For this review, take the finished solid that the model builds, in its own axes (mm). Give positions to 0.01 mm unless a question says otherwise; leave off trailing zeros. Order: outer loops, then holes, each group sorted by start corner. A loop starts at its lowest first (then second) coordinate and runs counter-clockwise, first axis right, second up. Notation, with made-up numbers: M 32.25,51 L 63.25,51 A15 cw 63.25,69 Z; hole C 0,44 d10. An arc over 180 degrees is marked long. Answer as CSV lines item,"result". Start each with the question number.
1. We need section B-B, the plane z = 8. Give the boundary of the cut face in (x, y), and give its area (3 significant figures).
2. For line 1 along Z through (x, y) = (30, 0.5); line 2 along X through (y, z) = (2.1, 31.5); line 3 along X through (y, z) = (2.35, -31.5), list the stretches that pass through material, from the lowest coordinate up.
3. We need section C-C, the plane z = -16.5. Give the boundary of the cut face in (x, y).
4. Clearance check with flat-ended pins moving along their axes: P1, Ø1.5, axis at y = 1.5, z = -32.5, coming from the +X side; P2, Ø1.8, axis at x = 43.75, z = 31.5, coming from the +Y side; P3, Ø1, axis at x = -29, y = 2, coming from the -Z side; P4, Ø0.9, axis at y = 1.5, z = 0.5, coming from the +X side. State where each tip first meets the part, or that it passes through.
5. We need section D-D, the plane y = 1.3. State how many separate pieces and enclosed holes the cut face has, and give its area (3 significant figures).
6. We need section A-A, the plane x = -43.25. Give the boundary of the cut face in (y, z).
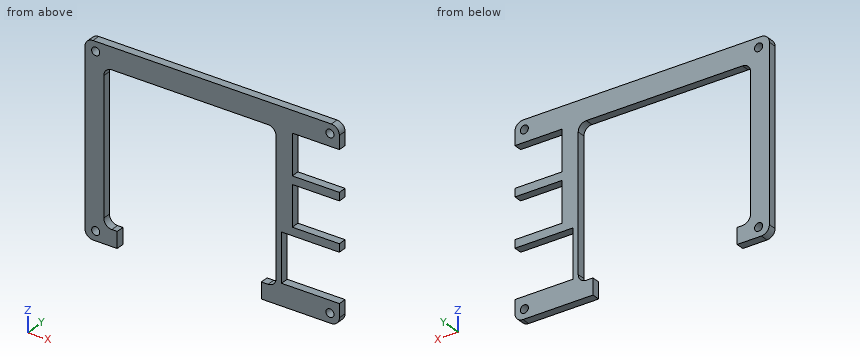
from build123d import *

# Parameters (mm, degrees)
SKETCH1_W           = 94.5
SKETCH1_H           = 70
BOSS_EXTRUDE1_DEPTH = 3
SKETCH3_R           = 1.5
CUT_EXTRUDE2_DEPTH  = 59.877521177
FILLET2_R           = 3
SKETCH5_W           = 64
SKETCH5_H           = 56
SKETCH5_W_2         = 53.5
SKETCH5_H_2         = 6
SKETCH5_W_3         = 21.5
SKETCH5_H_3         = 18
SKETCH5_W_4         = 17.5
SKETCH5_H_4         = 15
CUT_EXTRUDE3_DEPTH  = 59.877521177
FILLET3_R           = 3


with BuildPart() as part:
    # Sketch1 → Boss-Extrude1 (new body)
    with BuildSketch(Plane(origin=(0, 0, 0), x_dir=(1, 0, 0), z_dir=(0, 1, 0))):
        Rectangle(SKETCH1_W, SKETCH1_H)
    extrude(amount=BOSS_EXTRUDE1_DEPTH)

    # Sketch3 → Cut-Extrude2 (cut, through all)
    with BuildSketch(Plane(origin=(0, 3, 0), x_dir=(1, 0, 0), z_dir=(0, 1, 0))):
        with Locations(Location((43.75, 31.5, 0), (0, 0, 270))):
            Circle(SKETCH3_R)
        with Locations(Location((-43.25, 31.5, 0), (0, 0, 270))):
            Circle(SKETCH3_R)
        with Locations(Location((-43.25, -31.5, 0), (0, 0, 270))):
            Circle(SKETCH3_R)
        with Locations(Location((43.75, -31.5, 0), (0, 0, 270))):
            Circle(SKETCH3_R)
    extrude(amount=-CUT_EXTRUDE2_DEPTH, mode=Mode.SUBTRACT)

    # Fillet2
    fillet2_edges = [part.edges().sort_by_distance(p)[0] for p in [
        (47.25, 1.5, 35),
        (-47.25, 1.5, 35),
        (-47.25, 1.5, -35),
        (47.25, 1.5, -35),
    ]]
    fillet(fillet2_edges, radius=FILLET2_R)

    # Sketch5 → Cut-Extrude3 (cut, through all)
    with BuildSketch(Plane(origin=(0, 3, 0), x_dir=(1, 0, 0), z_dir=(0, 1, 0))):
        with Locations((-8.25, 1)):
            Rectangle(SKETCH5_W, SKETCH5_H)
        with Locations((-8.5, 32)):
            Rectangle(SKETCH5_W_2, SKETCH5_H_2)
        with Locations((36.5, 18)):
            Rectangle(SKETCH5_W_3, SKETCH5_H_3)
        with Locations((38.5, -1.5)):
            Rectangle(SKETCH5_W_4, SKETCH5_H_4)
        with Locations((38.5, -19.5)):
            Rectangle(SKETCH5_W_4, SKETCH5_H_4)
    extrude(amount=-CUT_EXTRUDE3_DEPTH, mode=Mode.SUBTRACT)

    # Fillet3
    fillet3_edges = [part.edges().sort_by_distance(p)[0] for p in [
        (-40.25, 1.5, 27),
        (-40.25, 1.5, -29),
        (23.75, 1.5, -29),
        (23.75, 1.5, 27),
    ]]
    fillet(fillet3_edges, radius=FILLET3_R)


solid = part.part
Result set:
1,outline,"M -47.25,0 L -40.25,0 L -40.25,3 L -47.25,3 Z; M 23.75,0 L 29.75,0 L 29.75,3 L 23.75,3 Z"
1,area,"39.0 mm2"
2,line 1,"-35 to -27, -9 to -6, 9 to 12, 27 to 35"
2,line 2,"-47.25 to -44.75, -41.75 to 42.25, 45.25 to 47.25"
2,line 3,"-47.25 to -44.75, -41.75 to -35.25, 18.25 to 42.25, 45.25 to 47.25"
3,outline,"M -47.25,0 L -40.25,0 L -40.25,3 L -47.25,3 Z; M 23.75,0 L 25.75,0 L 25.75,3 L 23.75,3 Z"
4,P1,"x = 47.25"
4,P2,"through"
4,P3,"z = 27"
4,P4,"x = 29.75"
5,separate pieces,"1"
5,enclosed holes,"4"
5,area,"1,770 mm2"
6,outline,"M 0,-35 L 3,-35 L 3,-33 L 0,-33 Z; M 0,-30 L 3,-30 L 3,30 L 0,30 Z; M 0,33 L 3,33 L 3,35 L 0,35 Z"
